Part model, mm, in its own coordinate system. Face numbers are marked on the shaded views. A direction names the side the tool comes from. Round coordinates to 2 decimals unless told otherwise and drop trailing zeros. Write each loop counter-clockwise with the first axis right and the second up, starting at its lowest first coordinate (ties: lowest second). Pieces come first, ordered by that corner, then holes.
```python
from build123d import *

# Parameters (mm, degrees)
CYLINDER_R                        = 10
CYLINDER_DEPTH                    = 250
CYLINDER_PITCH_ANGLE              = 90
REVOLVE_ONTO_SKETCH006_ROLL_ANGLE = 90
SKETCH003_R                       = 25
SKETCH003_R_2                     = 14
EXTRUDE003_DEPTH                  = 5
SKETCH005_R                       = 1.75
EXTRUDE005_DEPTH                  = 12
SKETCH004_R                       = 25
SKETCH004_R_2                     = 16.2
EXTRUDE004_DEPTH                  = 12
SKETCH002_R                       = 47
SKETCH002_R_2                     = 16.2
EXTRUDE002_DEPTH                  = 11
FUSION001_PLACEMENT_ANGLE         = 180


with BuildPart() as cylinder:
    # Cylinder → Cylinder (new body)
    with BuildSketch(Plane.XY):
        Circle(CYLINDER_R)
    extrude(amount=CYLINDER_DEPTH)


with BuildPart() as cylinder_1:
    # Cylinder pitch: moved
    add(cylinder.part.rotate(Axis((0, 0, 0), (0, 1, 0)), CYLINDER_PITCH_ANGLE))


with BuildPart() as cylinder_2:
    # Cylinder placement: moved
    add(cylinder_1.part.moved(Location((-125, 0, 15.25))))


with BuildPart() as cut001:
    # Sketch006 as drawn → Revolve (revolve)
    with BuildSketch(Plane.XY):
        Polygon((80, 27), (42.889, 80), (46.889, 80), (84, 27), (82, 0), (78, 0), align=None)
    revolve(axis=Axis((0, 0, 0), (0, 1, 0)))


with BuildPart() as cut001_1:
    # Revolve onto Sketch006 roll: moved
    add(cut001.part.rotate(Axis((0, 0, 0), (1, 0, 0)), REVOLVE_ONTO_SKETCH006_ROLL_ANGLE))


with BuildPart() as cut001_2:
    # Revolve onto Sketch006 placement: moved
    add(cut001_1.part)

    # Cut001: cut Cylinder
    add(cylinder_2.part, mode=Mode.SUBTRACT)


with BuildPart() as extrude003:
    # Sketch003 → Extrude003 (new body)
    with BuildSketch(Plane.XY):
        Circle(SKETCH003_R)
        Circle(SKETCH003_R_2, mode=Mode.SUBTRACT)
    extrude(amount=EXTRUDE003_DEPTH)


with BuildPart() as extrude003_1:
    # Extrude003 placement: moved
    add(extrude003.part.moved(Location((0, 0, 12))))


with BuildPart() as extrude005:
    # Sketch005 → Extrude005 (new body)
    with BuildSketch(Plane.XY):
        with Locations((-20, 0)):
            Circle(SKETCH005_R)
        with Locations((0, -20)):
            Circle(SKETCH005_R)
        with Locations((20, 0)):
            Circle(SKETCH005_R)
        with Locations((0, 20)):
            Circle(SKETCH005_R)
    extrude(amount=EXTRUDE005_DEPTH)


with BuildPart() as cut:
    # Sketch004 → Extrude004 (new body)
    with BuildSketch(Plane.XY):
        Circle(SKETCH004_R)
        Circle(SKETCH004_R_2, mode=Mode.SUBTRACT)
    extrude(amount=EXTRUDE004_DEPTH)

    # Cut: cut Extrude005
    add(extrude005.part, mode=Mode.SUBTRACT)


with BuildPart() as fusion001:
    # Sketch002 → Extrude002 (new body)
    with BuildSketch(Plane.XY):
        Circle(SKETCH002_R)
        Circle(SKETCH002_R_2, mode=Mode.SUBTRACT)
    extrude(amount=EXTRUDE002_DEPTH)


with BuildPart() as fusion001_1:
    # Extrude002 placement: moved
    add(fusion001.part.moved(Location((0, 0, 17))))

    # Fusion: union Extrude003, Cut
    add(extrude003_1.part)
    add(cut.part)


with BuildPart() as fusion001_2:
    # Fusion placement: moved
    add(fusion001_1.part.moved(Location((0, 0, 63))))

    # Fusion001: union Cut001
    add(cut001_2.part)


with BuildPart() as fusion001_3:
    # Fusion001 placement: moved
    add(fusion001_2.part.rotate(Axis((0, 0, 0), (1, 0, 0)), FUSION001_PLACEMENT_ANGLE))


solid = fusion001_3.part
```
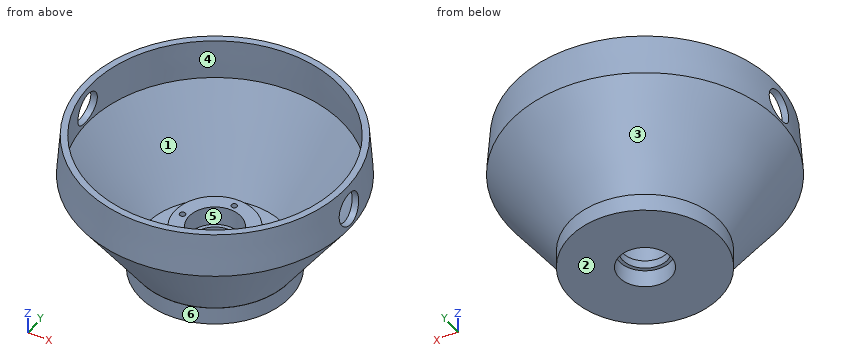
Q1. Cut at A-A on z = -65.5. Write the cut outline in (x, y).
Values follow:
outline: circle Ø114.08 at (0, 0); circle Ø50 at (0, 0); hole circle Ø106.08 at (0, 0); hole circle Ø3.5 at (-20, 0); hole circle Ø32.4 at (0, 0); hole circle Ø3.5 at (0, -20); hole circle Ø3.5 at (0, 20); hole circle Ø3.5 at (20, 0)
Q2. Cut at B-B on z = -36. Write the cut outline in (x, y).
Values follow:
outline: circle Ø155.4 at (0, 0); hole circle Ø147.4 at (0, 0)
Q3. Mould opens along X. For the marked faces 1, 2 and 3 say: +X half, -X half, draft (parallel to the pull), parting line (faces both ways), or undercut.
Values follow:
face 1: undercut
face 2: draft
face 3: parting line
Q4. Wall check: L1, parallel to Y at x = -20, z = -67.5; L2, parallel to X at y = 0, z = -83; L3, parallel to X at y = 0, z = -76.15. Give the ranges that are in metal, low to high.
Values follow:
L1: y = -51.92 to -47.61, -15 to -1.75, 1.75 to 15, 47.61 to 51.92
L2: x = -47 to -16.2, 16.2 to 47
L3: x = -49.58 to -45.58, -25 to -14, 14 to 25, 45.58 to 49.58
Q5. Drop flat-ended pins along their axis: pin 1 (1.8 mm diameter, centred on x = 0.5, y = -20.5, fed in from +Z); pin 2 (12 mm diameter, centred on y = -66.5, z = -12, fed in from -X); pin 3 (1.5 mm diameter, centred on x = -41.5, z = -22, fed in from +Y). Give the stop position or say it passes through.
Values follow:
pin 1: stops at z = -75
pin 2: stops at x = -56.69
pin 3: stops at y = 73.03
Q6. Which spindle directions (+Z, -Z, +X, -X, +Y, -Y) get a long thin tool onto all of the face, cutting with end or side? Do the marked faces 4, 5 and 6. Say none if no direction does.
Values follow:
face 4: none
face 5: +Z
face 6: -Z
